The listing builds one solid part. Answer for the finished solid, in the listing's coordinates (mm). Face numbers are marked on the shaded views. A direction names the side the tool comes from. Round coordinates to 2 decimals unless told otherwise and drop trailing zeros. Write each loop counter-clockwise with the first axis right and the second up, starting at its lowest first coordinate (ties: lowest second). Pieces come first, ordered by that corner, then holes. Notation, with made-up numbers: (60.25, -22.75) - (118.25, -22.75) arc R12 ccw to (118.25, -16.75) - close; hole circle Ø10 at (-22.75, 74.25). An arc over 180 degrees is marked (long way). Use a Markdown table: item, result. Add a question column.
1) A cutting plane is placed at B-B (x = 44.5). Give the vertices of the cut face in (y, z).
2) A tool of negligible diameter and unlimited length cuts with its end or side. For the marked faces 1, 2 and 3, from which of +Z, -Z, +X, -X, +Y, -Y can it reach the whole face along a straight path? Write none if from no direction.
3) A cutting plane is placed at A-A (x = 200). Give the vertices of the cut face in (y, z), then the cut area to 3 significant figures.
4) A cutting plane is placed at C-C (z = 0). State how many separate pieces and enclosed holes the cut face has, then the cut area to 3 significant figures.
5) A cutting plane is placed at D-D (y = 32). Give the vertices of the cut face in (x, z).
6) Find the intervals of material crossed by probe 1 along Z at (x, y) = (-101, 3.2); probe 2 along Z at (x, y) = (200, 52.05); probe 3 along Y at (x, z) = (71, -2), in increasing order. Write a range as from..to.
7) Each of these flat-tipped pins is pushed along its axis until it touches: P1, Ø1.2, axis at y = 52.5, z = 0, coming from the +X side; P2, Ø5, axis at x = 79, z = 5, coming from the -Y side; P3, Ø4, axis at y = 44, z = -1.5, coming from the +X side; P4, Ø11, axis at x = 200, z = 0, coming from the +Y side. Where does it stop, or does it pass through?
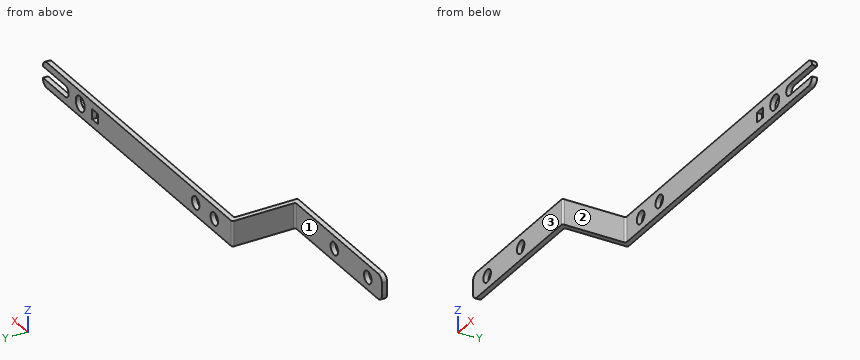
```python
from build123d import *

# Parameters (mm, degrees)
F2_DEPTH = 10
F3_R     = 5
F3_R_2   = 6
F3_W     = 8
F3_H     = 8
F4_DEPTH = 54.001
F5_R     = 5
F6_R     = 1.5


with BuildPart() as f2:
    # F1 (on Top) → F2 (new body, symmetric)
    with BuildSketch(Plane.XY):
        Polygon((0, 0), (0, 50), (250, 50), (250, 54), (-4, 54), (-4, 4), (-120, 4), (-120, 0), align=None)
    extrude(amount=F2_DEPTH, both=True)

    # F3 (on Front) → F4 (cut, through all)
    with BuildSketch(Plane.XZ):
        with Locations((-101, 0)):
            Circle(F3_R)
        with Locations((-56, 0)):
            Circle(F3_R)
        with Locations((20, 0)):
            Circle(F3_R)
        with Locations((45, 0)):
            Circle(F3_R)
        with Locations((200, 0)):
            Circle(F3_R_2)
        with BuildLine():
            ThreePointArc((220, -4.5), (223.1819805153, -3.1819805153), (224.5, 0))
            ThreePointArc((224.5, 0), (223.1819805153, 3.1819805153), (220, 4.5))
            ThreePointArc((220, 4.5), (215.5, 0), (220, -4.5))
        make_face()
        with BuildLine():
            ThreePointArc((220, 4.5), (223.1819805153, 3.1819805153), (224.5, 0))
            ThreePointArc((224.5, 0), (223.1819805153, -3.1819805153), (220, -4.5))
            Line((220, -4.5), (250, -4.5))
            Line((250, -4.5), (250, 4.5))
            Line((250, 4.5), (220, 4.5))
        make_face()
        with Locations((180, 0)):
            Rectangle(F3_W, F3_H)
    extrude(amount=-F4_DEPTH, mode=Mode.SUBTRACT)

    # F5
    f5_edges = [f2.edges().sort_by_distance(p)[0] for p in [
        (-120, 2, 10),
        (-120, 2, -10),
        (250, 52, -10),
        (250, 52, 10),
    ]]
    fillet(f5_edges, radius=F5_R)

    # F6
    f6_edges = [f2.edges().sort_by_distance(p)[0] for p in [
        (-4, 54, 0),
        (0, 50, 0),
        (0, 0, 0),
        (-4, 4, 0),
    ]]
    fillet(f6_edges, radius=F6_R)


solid = f2.part
```
Entries:
| question | item | result |
|---|---|---|
| 1 | outline | (50, -10) - (54, -10) - (54, -4.97) - (50, -4.97) - close; (50, 4.97) - (54, 4.97) - (54, 10) - (50, 10) - close |
| 2 | face 1 | +Z, -Z, -X, +Y |
| 2 | face 2 | +Z, -Z, +X, -Y |
| 2 | face 3 | +Z, -Z, +X, -X, -Y |
| 3 | outline | (50, -10) - (54, -10) - (54, -6) - (50, -6) - close; (50, 6) - (54, 6) - (54, 10) - (50, 10) - close |
| 3 | area | 32.0 mm² |
| 4 | separate pieces | 7 |
| 4 | enclosed holes | 0 |
| 4 | area | 1,300 mm² |
| 5 | outline | (-4, -10) - (0, -10) - (0, 10) - (-4, 10) - close |
| 6 | probe 1 | z = -10..-5, 5..10 |
| 6 | probe 2 | z = -10..-6, 6..10 |
| 6 | probe 3 | y = 50..54 |
| 7 | P1 | stops at x = 215.54 |
| 7 | P2 | stops at y = 50 |
| 7 | P3 | stops at x = 0 |
| 7 | P4 | passes through |
